The listing builds one solid part. Answer for the finished solid, in the listing's coordinates (mm). Face numbers are marked on the shaded views. A direction names the side the tool comes from. Coordinates: 2 decimals unless noted, no trailing zeros. Order: outer loops, then holes, each group sorted by start corner. A loop starts at its lowest first (then second) coordinate and runs counter-clockwise, first axis right, second up. Notation, with made-up numbers: (23.25, 76.5) -> (62.25, 76.5) arc R5 ccw to (62.25, 83.5) -> close; hole circle Ø7 at (-15, 76.5). An arc over 180 degrees is marked (long way). Write item = value, one per line.
Autodesk Inventor part; units mm, degrees
ref_plane "YZ Plane" through (0, 0, 0) normal (1, 0, 0) x (0, 1, 0)
ref_plane "XZ Plane" through (0, 0, 0) normal (0, 1, 0) x (-1, 0, 0)
ref_plane "XY Plane" through (0, 0, 0) normal (0, 0, 1) x (1, 0, 0)
sketch "Sketch1" plane through (0, 0, 0) normal (0, 0, 1) x (1, 0, 0)
  line L0 (0, 0) -> (9, 0)
  line L1 (9, 0) -> (9, 10.5)
  line L2 (9, 10.5) -> (0, 10.5)
  line L3 (0, 10.5) -> (0, 0)
  dimension "d0" = 9
  dimension "d1" = 10.5
extrude "Extrusion1" add sketch "Sketch1" along normal blind 17.4
sketch "Sketch2" plane through (0, 0, 17.4) normal (0, 0, 1) x (1, 0, 0)
  line L0 (9, 10.5) -> (0, 10.5) construction
  line L1 (4.5, 10.5) -> (4.5, 0) construction
  circle A0 centre (4.5, 5.5) radius 4
  point P0 (0, 0)
  dimension "d4" = 8
  dimension "d5" = 5
extrude "Extrusion2" add sketch "Sketch2" along normal blind 4.5
sketch "Sketch3" plane through (0, 0, 17.4) normal (0, 0, 1) x (1, 0, 0)
  line L0 (9, 10.5) -> (0, 10.5) construction
  line L1 (4.5, 10.5) -> (4.5, 0) construction
  line L2 (0, 0) -> (9, 0) construction
  line L3 (1.6586, 10.5) -> (0, 9.5141)
  line L4 (0, 10.5) -> (0, 0)
  line L5 (0, 9.5141) -> (0, 10.5)
  line L6 (0, 10.5) -> (1.6586, 10.5)
  line L7 (7.3414, 10.5) -> (9, 9.5141)
  line L8 (9, 9.5141) -> (9, 10.5)
  line L9 (9, 10.5) -> (7.3414, 10.5)
extrude "Extrusion3" cut sketch "Sketch3" against normal through all
properties part number "jack"
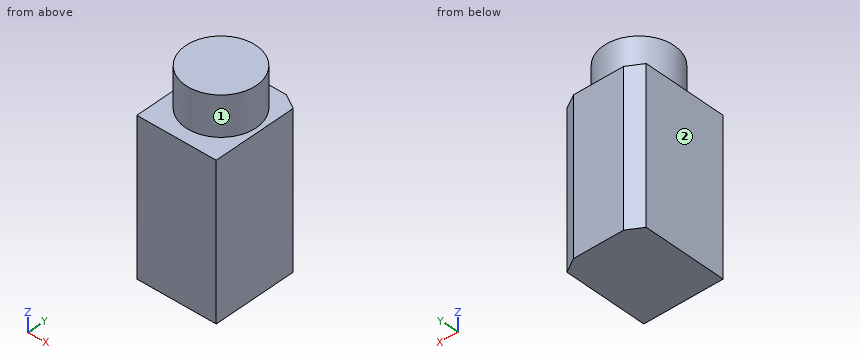
Q1. Section B-B, the plane x = 4.5 is taken. Give the vertices of the cut face in (y, z), plus the area to 3 significant figures.
The answers:
outline = (0, 0) -> (10.5, 0) -> (10.5, 17.4) -> (9.5, 17.4) -> (9.5, 21.9) -> (1.5, 21.9) -> (1.5, 17.4) -> (0, 17.4) -> close
area = 219 mm2
Q2. Section C-C, the plane z = 14.5 is taken. Give the vertices of the cut face in (x, y), plus the area to 3 significant figures.
The answers:
outline = (0, 0) -> (9, 0) -> (9, 9.51) -> (7.34, 10.5) -> (1.66, 10.5) -> (0, 9.51) -> close
area = 92.9 mm2
Q3. This flat-tipped pin is pushed along its axis until it touches: pin 1 Ø4 at (x, y) = (3, 6.5) entering from -Z. Where does it stop, or does it pass through?
The answers:
pin_1 = 0
Q4. Find the intervals of material crossed by line 1 along Z through (x, y) = (1.5, 1.25); line 2 along Y through (x, z) = (4.5, 17.5); line 3 along Y through (x, z) = (3.25, 17.5), in increasing order.
The answers:
line_1 = 0 to 17.4
line_2 = 1.5 to 9.5
line_3 = 1.7 to 9.3
Q5. A tool of negligible diameter and unlimited length cuts with its end or side. For the marked faces 1 and 2, from which of +Z, -Z, +X, -X, +Y, -Y can it reach the whole face along a straight path? Write none if from no direction.
The answers:
face_1 = +Z
face_2 = +Z, -Z, -X, +Y, -Y
Q6. Section D-D, the plane z = 20.25 is taken. Give the vertices of the cut face in (x, y), plus the area to 3 significant figures.
The answers:
outline = circle Ø8 at (4.5, 5.5)
area = 50.3 mm2
Q7. Section A-A, the plane y = 5.5 is taken. Give the vertices of the cut face in (x, z), plus the area to 3 significant figures.
The answers:
outline = (0, 0) -> (9, 0) -> (9, 17.4) -> (8.5, 17.4) -> (8.5, 21.9) -> (0.5, 21.9) -> (0.5, 17.4) -> (0, 17.4) -> close
area = 193 mm2
